Autodesk Inventor part; units mm, degrees
ref_plane "YZ Plane" through (0, 0, 0) normal (1, 0, 0) x (0, 1, 0)
ref_plane "XZ Plane" through (0, 0, 0) normal (0, 1, 0) x (-1, 0, 0)
ref_plane "XY Plane" through (0, 0, 0) normal (0, 0, 1) x (1, 0, 0)
sketch "Sketch1" plane through (0, 0, 0) normal (0, 0, 1) x (1, 0, 0)
  line L0 (0, 0) -> (118, 0)
  line L1 (118, 0) -> (118, 56)
  line L2 (118, 56) -> (0, 56)
  line L3 (0, 56) -> (0, 0)
  circle A0 centre (59, 28) radius 19.5
  circle A1 centre (38.415, 48.585) radius 2
  circle A2 centre (38.415, 7.415) radius 2
  circle A3 centre (79.585, 7.415) radius 2
  circle A4 centre (79.585, 48.585) radius 2
  dimension "width" = 118
  dimension "height" = 56
  dimension "d4" = 39
  dimension "d5" = 28
  dimension "d6" = 59
  dimension "d7" = 4
  dimension "d8" = 38.415
  dimension "d11" = 360
  dimension "d13" = 7.415
extrude "Extrusion2" add sketch "Sketch1" along normal blind 8
hole "Hole1" at (104, 28, 8) direction (0, 0, -1) diameter 6 end through all
hole "Hole2" at (14, 28, 8) direction (0, 0, -1) diameter 6 end through all
equation "\"d5\" = 0.5 * height"
equation "\"d6\" = 0.5 * width"
equation "\"d17\" = 0.5 * height"
equation "\"d26\" = 0.5 * height"
properties part number "support motor2"
Work out the finished part from the listing and answer in its coordinate system (mm). Give positions to 0.01 mm unless a question says otherwise; leave off trailing zeros. Loops run counter-clockwise (first coordinate to the right, second up) from the corner with the lowest first, then second, coordinate; pieces in that order, holes last. Notation, with made-up numbers: (64.5, -20.5) -> (75.5, -20.5) arc R29 cw to (75.5, 11.5) -> close; hole circle Ø1 at (4.25, 85). An arc over 180 degrees is marked (long way). Write item = value, one per line. Start each with the question number.
(1) Find section D-D on z = 3.75. Give the vertices of the cut face in (x, y) (3 decimals), and give its area (3 significant figures).
(2) Find the intervals of material crossed by probe 1 along X at (y, z) = (30, 7.75); probe 2 along X at (y, z) = (7, 1); probe 3 along Y at (x, z) = (39, 7), in increasing order. Write a range as from..to.
(3) The mould has two halves that part along Y. Classify faces 1 (the cylindrical face through (15.8, 30.4, 3.9)), 2 (the flat face through (58, 0, 4)), 3 (the flat face through (45, 47, 0)): +Y half, -Y half, draft (parallel to the pull), parting line (faces both ways), or undercut.
(4) Find section B-B on y = 20.5. Give the vertices of the cut face in (x, z).
(5) Find section C-C on y = 28. Give the vertices of the cut face in (x, z), and give its area (3 significant figures).
(6) Find section A-A on x = 59. Give the vertices of the cut face in (y, z).
From the geometry:
q1.outline = (0, 0) -> (118, 0) -> (118, 56) -> (0, 56) -> close; hole circle Ø6 at (14, 28); hole circle Ø4 at (38.415, 7.415); hole circle Ø4 at (38.415, 48.585); hole circle Ø39 at (59, 28); hole circle Ø4 at (79.585, 7.415); hole circle Ø4 at (79.585, 48.585); hole circle Ø6 at (104, 28)
q1.area = 5,310 mm^2
q2.probe_1 = 0..11.76, 16.24..39.6, 78.4..101.76, 106.24..118
q2.probe_2 = 0..36.46, 40.37..77.63, 81.54..118
q2.probe_3 = 0..5.5, 9.33..46.67, 50.5..56
q3.face_1 = undercut
q3.face_2 = -Y half
q3.face_3 = draft
q4.outline = (0, 0) -> (41, 0) -> (41, 8) -> (0, 8) -> close; (77, 0) -> (118, 0) -> (118, 8) -> (77, 8) -> close
q5.outline = (0, 0) -> (11, 0) -> (11, 8) -> (0, 8) -> close; (17, 0) -> (39.5, 0) -> (39.5, 8) -> (17, 8) -> close; (78.5, 0) -> (101, 0) -> (101, 8) -> (78.5, 8) -> close; (107, 0) -> (118, 0) -> (118, 8) -> (107, 8) -> close
q5.area = 536 mm^2
q6.outline = (0, 0) -> (8.5, 0) -> (8.5, 8) -> (0, 8) -> close; (47.5, 0) -> (56, 0) -> (56, 8) -> (47.5, 8) -> close
